```python
from build123d import *

# Parameters (mm, degrees)
CUT_EXTRUDE_1_DEPTH = 1.5
CHAMFER_1_SIZE      = 0.2
CHAMFER_1_SIZE2     = 0.146618763


with BuildPart() as part:
    # 草图1 → 旋转5 (revolve)
    with BuildSketch(Plane(origin=(0, 0, 0), x_dir=(1, 0, 0), z_dir=(0, 1, 0))):
        Polygon((-2.008479615, -0.003832891), (-0.008479615, -0.003832891), (-0.008479615, -6.003832891), (-1.008479615, -6.003832891), (-1.008479615, -1.757110008), align=None)
    revolve(axis=Axis((-0.008479615, 0, 0.003832891), (0, 0, 1)))

    # 草图2 → 切除-拉伸1 (cut)
    with BuildSketch(Plane.XY.offset(0.003832891)):
        Polygon((0.857545789, 0), (0.424533087, 0.75), (-0.441492317, 0.75), (-0.874505018, 0), (-0.441492317, -0.75), (0.424533087, -0.75), align=None)
    extrude(amount=CUT_EXTRUDE_1_DEPTH, mode=Mode.SUBTRACT)

    # 倒角1
    chamfer_1_edges = [part.edges().sort_by_distance(p)[0] for p in [
        (1.991520385, 0, 0.003832891),
    ]]
    chamfer_1_side = [part.faces().sort_by_distance(p)[0] for p in [
        (1.491520385, 0, 0.880471449),
    ]]
    chamfer(chamfer_1_edges, length=CHAMFER_1_SIZE, length2=CHAMFER_1_SIZE2, reference=chamfer_1_side[0])


solid = part.part
```
Geometry check sheet. Reference: the model listing, model coordinates, mm. A direction names the side the tool comes from. Round coordinates to 2 decimals unless told otherwise and drop trailing zeros. Order: outer loops, then holes, each group sorted by start corner. A loop starts at its lowest first (then second) coordinate and runs counter-clockwise, first axis right, second up. Notation, with made-up numbers: (22, 62) -> (67, 62) arc R6 ccw to (67, 70) -> close; hole circle Ø7 at (30, 26). An arc over 180 degrees is marked (long way). Return JSON: item names as keys, results as strings. Group by question number.
Q1. Release check for a two-part mould opening along X. For faces 1 (the flat face through (0, 1, 0.004)), 2 (the flat face through (0, -0.75, 1)), 3 (the cylindrical face through (0, 1, 4)) record: released by +X, released by -X, zero draft, split by the parting line, or undercut.
Q2. Section check A-A, the plane z = 2.7. Record the boundary of the cut face in (x, y), plus the area to 3 significant figures.
Q3. Tool access check on faces 4 (the flat face through (0, 0, 1.504)), 5 (the flat face through (0, 0, 6.004)). Record the directions out of +Z, -Z, +X, -X, +Y, -Y that give a thin tool (end or side, any length) a straight path to the whole face; none if there is none.
Q4. Material ranges on probe 1 along Y at (x, z) = (-0.75, 0.7); probe 2 along X at (y, z) = (-0.45, 2.95); probe 3 along Y at (x, z) = (0.7, 5), recorded low to high. Write a range as from..to.
Q5. Gauge pin test, flat end, axial feed: pin 1 (1.5 mm diameter, centred on x = 0, z = 4, fed in from -Y). Record the tip position at first contact, or that the pin passes through.
Numbers:
{
 "1": {"face 1": "zero draft", "face 2": "undercut", "face 3": "split by the parting line"},
 "2": {"outline": "circle Ø2 at (-0.01, 0)", "area": "3.14 mm^2"},
 "3": {"face 4": "-Z", "face 5": "+Z, +X, -X, +Y, -Y"},
 "4": {"probe 1": "-1.42..-0.22, 0.22..1.42", "probe 2": "-0.9..0.88", "probe 3": "-0.71..0.71"},
 "5": {"pin 1": "y = -1"}
}
